Drawing for the job (mm, zero at the part's lowest x, y, z). Round coordinates to 2 decimals unless told otherwise and drop trailing zeros. Order: outer loops, then holes, each group sorted by start corner. A loop starts at its lowest first (then second) coordinate and runs counter-clockwise, first axis right, second up. Notation, with made-up numbers: (-8, 2) - (32, 2) arc R6 ccw to (32, 9) - close; hole circle Ø9 at (39, 36.25). An arc over 180 degrees is marked (long way). Answer as a JSON object with one key per item and string values.
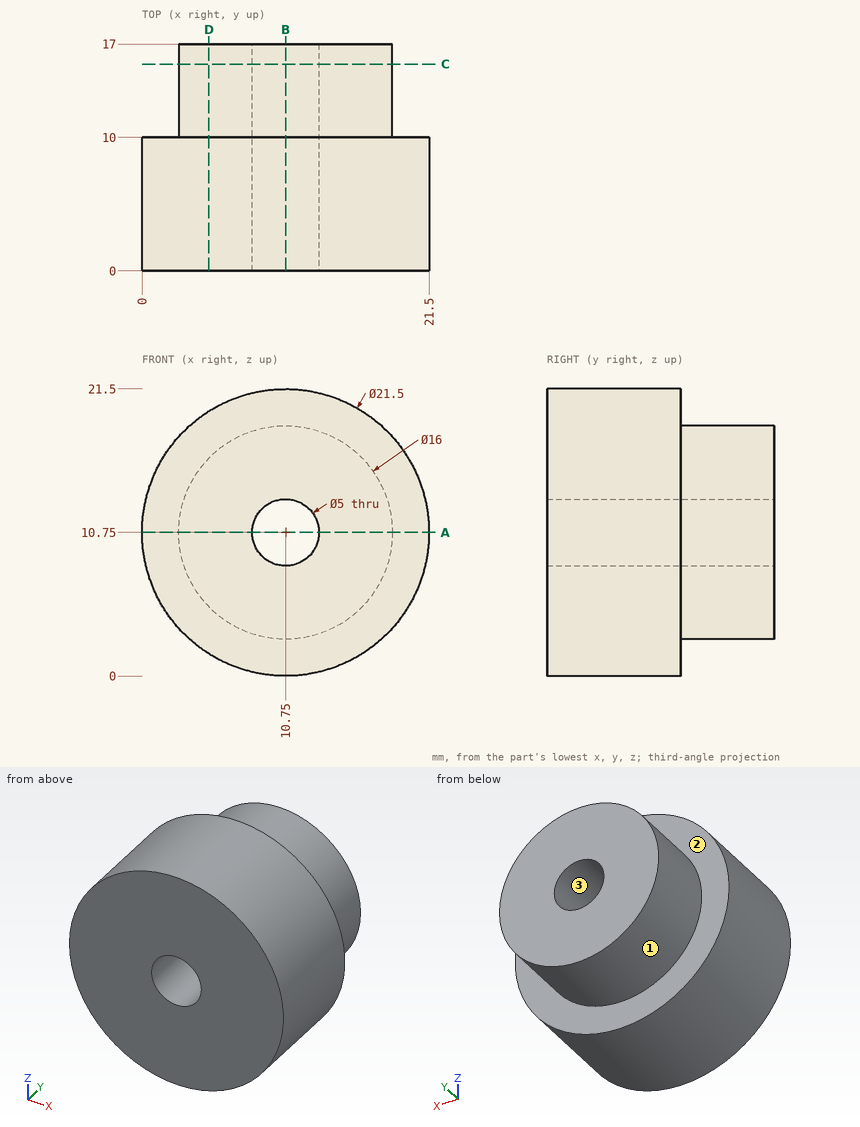
Item 1: Cut at B-B (x = 10.75). Write the cut outline in (y, z), plus the area to 3 significant figures.
Taken from the geometry:
{"outline": "(0, 0) - (10, 0) - (10, 2.75) - (17, 2.75) - (17, 8.25) - (0, 8.25) - close; (0, 13.25) - (17, 13.25) - (17, 18.75) - (10, 18.75) - (10, 21.5) - (0, 21.5) - close", "area": "242 mm2"}
Item 2: Cut at C-C (y = 15.5). Write the cut outline in (x, z).
Taken from the geometry:
{"outline": "circle Ø16 at (10.75, 10.75); hole circle Ø5 at (10.75, 10.75)"}
Item 3: Cut at A-A (z = 10.75). Write the cut outline in (x, y).
Taken from the geometry:
{"outline": "(0, 0) - (8.25, 0) - (8.25, 17) - (2.75, 17) - (2.75, 10) - (0, 10) - close; (13.25, 0) - (21.5, 0) - (21.5, 10) - (18.75, 10) - (18.75, 17) - (13.25, 17) - close"}
Item 4: Cut at D-D (x = 5). Write the cut outline in (y, z), plus the area to 3 significant figures.
Taken from the geometry:
{"outline": "(0, 1.67) - (10, 1.67) - (10, 5.19) - (17, 5.19) - (17, 16.31) - (10, 16.31) - (10, 19.83) - (0, 19.83) - close", "area": "260 mm2"}
Item 5: Probe L1, parallel to Z at x = 10.75, y = 9.75; L2, parallel to Z at x = 10.75, y = 13.25; L3, parallel to Y at x = 15.25, z = 3.5. List the from-to ranges inside material, lowest first. Write a range as from..to.
Taken from the geometry:
{"L1": "0..8.25, 13.25..21.5", "L2": "2.75..8.25, 13.25..18.75", "L3": "0..10"}
Item 6: Drop flat-ended pins along their axis: P1, Ø5, axis at y = 9, z = 19.5, coming from the +X side; P2, Ø1.5, axis at y = 14, z = 4.5, coming from the +X side; P3, Ø5, axis at x = 10, y = 14.5, coming from the +Z side. Give the stop position or say it passes through.
Taken from the geometry:
{"P1": "x = 19.5", "P2": "x = 16.56", "P3": "z = 18.75"}
Item 7: Two-plate mould, pull along X, no slides. Class the marked faces 1, 2 and 3: pulls with the +X half, pulls with the -X half, needs draft (parallel to the pull), parting line crosses it, or undercut.
Taken from the geometry:
{"face 1": "parting line crosses it", "face 2": "needs draft", "face 3": "undercut"}
